Work out the finished part from the listing and answer in its coordinate system (mm). A direction names the side the tool comes from. Give positions to 0.01 mm unless a question says otherwise; leave off trailing zeros. Order: outer loops, then holes, each group sorted by start corner. A loop starts at its lowest first (then second) coordinate and runs counter-clockwise, first axis right, second up.
```python
from build123d import *

# Parameters (mm, degrees)
CROQUIS1_W              = 471.25
CROQUIS1_H              = 55
SALIENTE_EXTRUIR1_DEPTH = 4
CROQUIS2_W              = 471.25
CROQUIS2_H              = 4
SALIENTE_EXTRUIR2_DEPTH = 55
REDONDEO1_R             = 3
REDONDEO2_R             = 1.5


with BuildPart() as part:
    # Croquis1 → Saliente-Extruir1 (new body)
    with BuildSketch(Plane.XY):
        Rectangle(CROQUIS1_W, CROQUIS1_H)
    extrude(amount=SALIENTE_EXTRUIR1_DEPTH)

    # Croquis2 → Saliente-Extruir2 (add)
    with BuildSketch(Plane(origin=(0, 0, 0), x_dir=(-1, 0, 0), z_dir=(0, 0, -1))):
        with Locations((0, -25.5)):
            Rectangle(CROQUIS2_W, CROQUIS2_H)
    extrude(amount=SALIENTE_EXTRUIR2_DEPTH)

    # Redondeo1
    redondeo1_edges = [part.edges().sort_by_distance(p)[0] for p in [
        (0, -23.5, 0),
    ]]
    fillet(redondeo1_edges, radius=REDONDEO1_R)

    # Redondeo2
    redondeo2_edges = [part.edges().sort_by_distance(p)[0] for p in [
        (0, -27.5, 4),
    ]]
    fillet(redondeo2_edges, radius=REDONDEO2_R)


solid = part.part
```
1. Straight lines are drawn through the part: probe 1 along Z at (x, y) = (-186, 22.5); probe 2 along Y at (x, z) = (171.5, -31); probe 3 along Z at (x, y) = (25, -21.5). For each, find the intervals that lie inside material, in ascending order.
Findings below:
probe 1: z = 0 to 4
probe 2: y = -27.5 to -23.5
probe 3: z = -0.17 to 4
2. The part is cut by section A-A (x = 51.5). Write down the section's boundary in (y, z).
Findings below:
outline: (-27.5, -55) - (-23.5, -55) - (-23.5, -3) arc R3 cw to (-20.5, 0) - (27.5, 0) - (27.5, 4) - (-26, 4) arc R1.5 ccw to (-27.5, 2.5) - close
3. The part is cut by section B-B (z = -49). Write down the section's boundary in (x, y) (3 decimals).
Findings below:
outline: (-235.625, -27.5) - (235.625, -27.5) - (235.625, -23.5) - (-235.625, -23.5) - close
4. The part is cut by section C-C (y = 1.5). Write down the section's boundary in (x, z) (3 decimals).
Findings below:
outline: (-235.625, 0) - (235.625, 0) - (235.625, 4) - (-235.625, 4) - close
5. Which of the six approach directions +Z, -Z, +X, -X, +Y, -Y give full straight-line access (tool end or side, diameter ignored) to faces 1 (the face through (3, -23.5, -29)), 2 (the face through (-235.625, -25, -12))?
Findings below:
face 1: -Z, +X, -X, +Y
face 2: +Z, -Z, -X, +Y, -Y
6. Given P1, Ø14.5, axis at x = -107.5, y = -1, coming from the -Z side; P2, Ø1.5, axis at x = 179.5, z = -23, coming from the +Y side; P3, Ø6, axis at y = -5.5, z = -2, coming from the -X side (3 decimals), each flat-ended and moving along its own axis, determine where each tip first touches the part or whether it passes through.
Findings below:
P1: stops at z = 0
P2: stops at y = -23.5
P3: stops at x = -235.625
